```python
from build123d import *

# Parameters (mm, degrees)
SKETCH1_W           = 12.7
SKETCH1_H           = 12.7
BOSS_EXTRUDE1_DEPTH = 300
SHELL18_T           = -1
SKETCH2_R           = 2
CUT_EXTRUDE1_DEPTH  = 30
SKETCH3_R           = 2
CUT_EXTRUDE2_DEPTH  = 20


with BuildPart() as part:
    # Sketch1 → Boss-Extrude1 (new body)
    with BuildSketch(Plane.XY):
        with Locations((0.433911759, -1.30095226)):
            Rectangle(SKETCH1_W, SKETCH1_H)
    extrude(amount=BOSS_EXTRUDE1_DEPTH)

    # Shell18
    shell18_openings = [part.faces().sort_by_distance(p)[0] for p in [
        (0.433911759, -1.30095226, 300),
        (0.433911759, -1.30095226, 0),
    ]]
    offset(amount=SHELL18_T, openings=shell18_openings, kind=Kind.INTERSECTION)

    # Sketch2 → Cut-Extrude1 (cut)
    with BuildSketch(Plane(origin=(0, 5.04904774, 0), x_dir=(1, 0, 0), z_dir=(0, 1, 0))):
        with Locations((0.433911759, -10.040040702)):
            Circle(SKETCH2_R)
        with Locations((0.433911759, -21.34849815)):
            Circle(SKETCH2_R)
    extrude(amount=-CUT_EXTRUDE1_DEPTH, mode=Mode.SUBTRACT)

    # Sketch3 → Cut-Extrude2 (cut)
    with BuildSketch(Plane(origin=(0, 5.04904774, 0), x_dir=(1, 0, 0), z_dir=(0, 1, 0))):
        with Locations((0.433911759, -336)):
            Circle(SKETCH3_R)
        with Locations((0.433911759, -316)):
            Circle(SKETCH3_R)
    extrude(amount=-CUT_EXTRUDE2_DEPTH, mode=Mode.SUBTRACT)


solid = part.part
```
Source: CAD feature listing. Evaluate the final solid. Frame: model axes, mm. A direction names the side the tool comes from. Round coordinates to 2 decimals unless told otherwise and drop trailing zeros. Write each loop counter-clockwise with the first axis right and the second up, starting at its lowest first coordinate (ties: lowest second). Pieces come first, ordered by that corner, then holes. Notation, with made-up numbers: M 19.25,89.25 L 43.25,89.25 A25 ccw 43.25,109.25 Z; hole C 28.25,8.25 d6. An arc over 180 degrees is marked long. Answer as a JSON object with one key per item and string values. Group by question number.
(1) Mould query, pull axis X, two halves, no side actions, for faces 1 (the flat face through (6.784, -1, 148)), 2 (the flat face through (0, 5.049, 148)), 3 (the flat face through (-4.916, -1, 148)), 4 (the flat face through (5.784, -1, 148)). Classes: +X half, -X half, draft (parallel to the pull), parting line (faces both ways), or undercut.
(2) Section query B-B on y = 1.75. Output: boundary loops of the cut face in (x, z), then the cut area to 3 significant figures.
(3) Reachability of faces 5 (the flat face through (6, -1, 300)), 6 (the flat face through (0, 4.049, 148)) from +Z, -Z, +X, -X, +Y, -Y: full face, straight path, thin tool, end or side. Return the list, or none.
(4) Ray query, line 1 (Y direction, x = 2.75, z = 118.5); line 2 (X direction, y = 0.25, z = 67). Return the intervals inside material, ascending. Write a range as [from, to].
(5) Section query A-A on z = 128. Output: boundary loops of the cut face in (x, y), then the cut area to 3 significant figures.
Computed values:
{
 "1": {"face 1": "+X half", "face 2": "draft", "face 3": "undercut", "face 4": "undercut"},
 "2": {"outline": "M -5.92,0 L -4.92,0 L -4.92,300 L -5.92,300 Z; M 5.78,0 L 6.78,0 L 6.78,300 L 5.78,300 Z", "area": "600 mm^2"},
 "3": {"face 5": "+Z, +X, -X, +Y, -Y", "face 6": "+Z, -Z"},
 "4": {"line 1": "[-7.65, -6.65], [4.05, 5.05]", "line 2": "[-5.92, -4.92], [5.78, 6.78]"},
 "5": {"outline": "M -5.92,-7.65 L 6.78,-7.65 L 6.78,5.05 L -5.92,5.05 Z; hole M -4.92,-6.65 L 5.78,-6.65 L 5.78,4.05 L -4.92,4.05 Z", "area": "46.8 mm^2"}
}
